```python
from build123d import *

# Parameters (mm, degrees)
SKETCH1_W           = 40
SKETCH1_H           = 40
BOSS_EXTRUDE1_DEPTH = 40
CUT_EXTRUDE1_DEPTH  = 40
SKETCH3_W           = 20
SKETCH3_H           = 10
CUT_EXTRUDE2_DEPTH  = 40


with BuildPart() as part:
    # Sketch1 → Boss-Extrude1 (new body)
    with BuildSketch(Plane.XY):
        with Locations((20, 20)):
            Rectangle(SKETCH1_W, SKETCH1_H)
    extrude(amount=BOSS_EXTRUDE1_DEPTH)

    # Sketch2 → Cut-Extrude1 (cut)
    with BuildSketch(Plane.XY.offset(40)):
        Polygon((0, 40), (20, 40), (0, 0), align=None)
    extrude(amount=-CUT_EXTRUDE1_DEPTH, mode=Mode.SUBTRACT)

    # Sketch3 → Cut-Extrude2 (cut)
    with BuildSketch(Plane.XZ):
        with Locations((10, 5)):
            Rectangle(SKETCH3_W, SKETCH3_H)
        Polygon((40, 0), (20, 10), (20, 0), align=None)
        with Locations((10, 35)):
            Rectangle(SKETCH3_W, SKETCH3_H)
        Polygon((20, 40), (20, 30), (40, 40), align=None)
    extrude(amount=-CUT_EXTRUDE2_DEPTH, mode=Mode.SUBTRACT)


solid = part.part
```
Read the model definition and answer for the solid it produces. Units are mm, in the model's axes. A direction names the side the tool comes from. Give positions to 0.01 mm unless a question says otherwise; leave off trailing zeros. Write each loop counter-clockwise with the first axis right and the second up, starting at its lowest first coordinate (ties: lowest second). Pieces come first, ordered by that corner, then holes. Notation, with made-up numbers: (37.25, 62) -> (70.25, 62) arc R14 cw to (70.25, 82) -> close; hole circle Ø11 at (77.25, 31.5). An arc over 180 degrees is marked (long way). Answer as a JSON object with one key per item and string values.
1) Straight lines are drawn through the part: probe 1 along Z at (x, y) = (14, 17); probe 2 along Y at (x, z) = (15, 11.5); probe 3 along X at (y, z) = (6.5, 28). For each, find the intervals that lie inside material, in ascending order. Write a range as from..to.
Findings below:
{"probe 1": "z = 10..30", "probe 2": "y = 0..30", "probe 3": "x = 3.25..40"}
2) Section D-D on y = 16 is taken. Write down the section's boundary in (x, z), then the cut area to 3 significant figures.
Findings below:
{"outline": "(8, 10) -> (20, 10) -> (40, 0) -> (40, 40) -> (20, 30) -> (8, 30) -> close", "area": "840 mm^2"}
3) For a pull along Z with two mould halves and no side action, classify faces 3 (the flat face through (14, 11, 10)), 4 (the flat face through (32, 40, 20)), 5 (the flat face through (30, 20, 35)) as pulls with the +Z half, pulls with the -Z half, needs draft (parallel to the pull), parting line crosses it, or undercut.
Findings below:
{"face 3": "pulls with the -Z half", "face 4": "needs draft", "face 5": "pulls with the +Z half"}
4) Flat-ended cylindrical pins translate along their axes: pin 1 Ø22 at (x, y) = (8.5, 18) entering from +Z; pin 2 Ø22 at (x, y) = (15, 18.5) entering from -Z; pin 3 Ø8 at (x, y) = (29, 17) entering from -Z; pin 4 Ø6 at (x, z) = (17.5, 19) entering from -Y. Find the tip coordinate at first contact, or state that the pin passes through.
Findings below:
{"pin 1": "stops at z = 30", "pin 2": "stops at z = 7", "pin 3": "stops at z = 3.5", "pin 4": "stops at y = 0"}
5) Section B-B on z = 36 is taken. Write down the section's boundary in (x, y), then the cut area to 3 significant figures.
Findings below:
{"outline": "(32, 0) -> (40, 0) -> (40, 40) -> (32, 40) -> close", "area": "320 mm^2"}
6) Section A-A on y = 7.5 is taken. Write down the section's boundary in (x, z).
Findings below:
{"outline": "(3.75, 10) -> (20, 10) -> (40, 0) -> (40, 40) -> (20, 30) -> (3.75, 30) -> close"}
7) A tool of negligible diameter and unlimited length cuts with its end or side. For faces 1 (the flat face through (40, 20, 20)), 2 (the flat face through (14, 11, 30)), from which of +Z, -Z, +X, -X, +Y, -Y can it reach the whole face along a straight path? Write none if from no direction.
Findings below:
{"face 1": "+Z, -Z, +X, +Y, -Y", "face 2": "+Z, -X, +Y, -Y"}
8) Section C-C on x = 32.5 is taken. Write down the section's boundary in (y, z), then the cut area to 3 significant figures.
Findings below:
{"outline": "(0, 3.75) -> (40, 3.75) -> (40, 36.25) -> (0, 36.25) -> close", "area": "1,300 mm^2"}
